For this review, take the finished solid that the model builds, in its own axes (mm). A direction names the side the tool comes from. Give positions to 0.01 mm unless a question says otherwise; leave off trailing zeros. Write each loop counter-clockwise with the first axis right and the second up, starting at its lowest first coordinate (ties: lowest second). Pieces come first, ordered by that corner, then holes.
1) We need section D-D on x = 2.5. Give the boundary of the cut face in (y, z), and give its area (3 significant figures).
2) Draft analysis for pull direction X (two halves, no side actions). For faces 3 (the face through (-9.613, 3.514, 23.186)), 4 (the face through (-27.07, 2.28, 27)), 5 (the face through (0, 3, 28.5)), state which applies: pulls with the +X half, pulls with the -X half, needs draft (parallel to the pull), parting line crosses it, or undercut.
3) We need section B-B on z = 18. Give the boundary of the cut face in (x, y).
4) We need section C-C on y = 3.5. Give the number of separate pieces and of enclosed holes in the cut face, and give its area (3 significant figures).
5) We need section A-A on x = 22. Give the boundary of the cut face in (y, z).
6) For P1, Ø6.5, axis at x = 23.5, z = -23.5, coming from the +Y side, flat-tipped, find the tip position at first contact; note if it passes through.
7) Machinability: for faces 1 (the face through (15.88, 1.27, -17.32)), 2 (the face through (22.4, 2.5, -7.6)), which of the approach directions +Z, -Z, +X, -X, +Y, -Y give a long, thin tool a straight path to every point of the face, cutting with its end or side? Answer none if there is none.
8) Wall thickness on line 1 along X through (y, z) = (1.15, 0); line 2 along X through (y, z) = (3.55, 15.5); line 3 along Y through (x, z) = (-5, 26.5): over which ranges is each line inside the solid? List them lowest first.
from build123d import *

# Parameters (mm, degrees)
SKETCH1_W                = 57
SKETCH1_H                = 57
BOSS_EXTRUDE1_DEPTH      = 4.5
FILLET1_R                = 5
SKETCH2_R                = 2.5
SKETCH2_R_2              = 1.7
CUT_EXTRUDE1_DEPTH       = 41.555517504
BOSS_EXTRUDE2_DEPTH      = 1
FILLET2_R                = 0.2
SKETCH4_R                = 23.5
CUT_EXTRUDE2_DEPTH       = 41.555517504
SKETCH4_3_R              = 25.1
SKETCH4_3_R_2            = 23.5
CUT_EXTRUDE3_DEPTH       = 2
CUT_EXTRUDE4_DEPTH       = 1.1
CIRPATTERN1_COUNT        = 4
FILLET2_OF_CIRPATTERN1_R = 0.2


with BuildPart() as part:
    # Sketch1 → Boss-Extrude1 (new body)
    with BuildSketch(Plane(origin=(0, 0, 0), x_dir=(1, 0, 0), z_dir=(0, 1, 0))):
        Rectangle(SKETCH1_W, SKETCH1_H)
    extrude(amount=BOSS_EXTRUDE1_DEPTH)

    # Fillet1
    fillet1_edges = [part.edges().sort_by_distance(p)[0] for p in [
        (-28.5, 2.25, -28.5),
        (28.5, 2.25, -28.5),
        (28.5, 2.25, 28.5),
        (-28.5, 2.25, 28.5),
    ]]
    fillet(fillet1_edges, radius=FILLET1_R)

    # Sketch2 → Cut-Extrude1 (cut, through all)
    with BuildSketch(Plane(origin=(0, 4.5, 0), x_dir=(1, 0, 0), z_dir=(0, 1, 0))):
        with Locations(Location((-23.5, 23.5, 0), (0, 0, 270))):
            Circle(SKETCH2_R)
        with Locations(Location((-15.5, 25, 0), (0, 0, 270))):
            Circle(SKETCH2_R_2)
    cut_extrude1 = extrude(amount=-CUT_EXTRUDE1_DEPTH, mode=Mode.SUBTRACT)

    # Sketch3 → Boss-Extrude2 (add)
    with BuildSketch(Plane(origin=(0, 4.5, 0), x_dir=(1, 0, 0), z_dir=(0, 1, 0))):
        Polygon((11, 27.5), (-11, 27.5), (-12, 28.5), (12, 28.5), align=None)
    boss_extrude2 = extrude(amount=BOSS_EXTRUDE2_DEPTH)

    # Fillet2
    fillet2_edges = [part.edges().sort_by_distance(p)[0] for p in [
        (0, 5.5, -27.5),
    ]]
    fillet(fillet2_edges, radius=FILLET2_R)

    # Sketch4 → Cut-Extrude2 (cut, through all)
    with BuildSketch(Plane(origin=(0, 4.5, 0), x_dir=(1, 0, 0), z_dir=(0, 1, 0))):
        with Locations(Location((0, 0, 0), (0, 0, 270))):
            Circle(SKETCH4_R)
    extrude(amount=-CUT_EXTRUDE2_DEPTH, mode=Mode.SUBTRACT)

    # Sketch4_3 → Cut-Extrude3 (cut)
    with BuildSketch(Plane(origin=(0, 4.5, 0), x_dir=(1, 0, 0), z_dir=(0, 1, 0))):
        with Locations(Location((0, 0, 0), (0, 0, 270))):
            Circle(SKETCH4_3_R)
        with Locations(Location((0, 0, 0), (0, 0, 270))):
            Circle(SKETCH4_3_R_2, mode=Mode.SUBTRACT)
    extrude(amount=-CUT_EXTRUDE3_DEPTH, mode=Mode.SUBTRACT)

    # Sketch5 → Cut-Extrude4 (cut)
    with BuildSketch(Plane.XZ):
        Polygon((-11, -27.5), (11, -27.5), (12, -28.5), (-12, -28.5), align=None)
    cut_extrude4 = extrude(amount=-CUT_EXTRUDE4_DEPTH, mode=Mode.SUBTRACT)

    # CirPattern1: Cut-Extrude1, Boss-Extrude2, Cut-Extrude4 ×4 about axis
    cirpattern1_axis = Axis((0, 0, 0), (0, 1, 0))
    add([cut_extrude1.rotate(cirpattern1_axis, i * 360 / CIRPATTERN1_COUNT) for i in range(1, CIRPATTERN1_COUNT)], mode=Mode.SUBTRACT)
    add([boss_extrude2.rotate(cirpattern1_axis, i * 360 / CIRPATTERN1_COUNT) for i in range(1, CIRPATTERN1_COUNT)])
    add([cut_extrude4.rotate(cirpattern1_axis, i * 360 / CIRPATTERN1_COUNT) for i in range(1, CIRPATTERN1_COUNT)], mode=Mode.SUBTRACT)

    # Fillet2 of CirPattern1
    fillet2_of_cirpattern1_edges = [part.edges().sort_by_distance(p)[0] for p in [
        (-27.5, 5.5, 0),
        (0, 5.5, 27.5),
        (27.5, 5.5, 0),
    ]]
    fillet(fillet2_of_cirpattern1_edges, radius=FILLET2_OF_CIRPATTERN1_R)


solid = part.part
Results list:
1. outline: (0, -27.5) - (1.1, -27.5) - (1.1, -28.5) - (5.5, -28.5) - (5.5, -27.7) arc R0.2 ccw to (5.3, -27.5) - (4.5, -27.5) - (4.5, -24.98) - (2.5, -24.98) - (2.5, -23.37) - (0, -23.37) - close; (0, 23.37) - (2.5, 23.37) - (2.5, 24.98) - (4.5, 24.98) - (4.5, 27.5) - (5.3, 27.5) arc R0.2 ccw to (5.5, 27.7) - (5.5, 28.5) - (1.1, 28.5) - (1.1, 27.5) - (0, 27.5) - close
1. area: 39.5 mm2
2. face 3: undercut
2. face 4: pulls with the -X half
2. face 5: needs draft
3. outline: (-28.5, 0) - (-15.11, 0) - (-15.11, 2.5) - (-17.49, 2.5) - (-17.49, 4.5) - (-28.5, 4.5) - close; (15.11, 0) - (28.5, 0) - (28.5, 4.5) - (17.49, 4.5) - (17.49, 2.5) - (15.11, 2.5) - close
4. separate pieces: 1
4. enclosed holes: 9
4. area: 1,130 mm2
5. outline: (0, -28.5) - (4.5, -28.5) - (4.5, -25.5) - (0, -25.5) - close; (0, -21.5) - (4.5, -21.5) - (4.5, -12.08) - (2.5, -12.08) - (2.5, -8.26) - (0, -8.26) - close; (0, 8.26) - (2.5, 8.26) - (2.5, 12.08) - (4.5, 12.08) - (4.5, 21.5) - (0, 21.5) - close; (0, 25.5) - (4.5, 25.5) - (4.5, 28.5) - (0, 28.5) - close
6. P1: stops at y = 4.5
7. face 1: +Y, -Y
7. face 2: +Y
8. line 1: x = -28.5 to -23.5, 23.5 to 28.5
8. line 2: x = -28.5 to -26.7, -23.3 to -19.74, 19.74 to 28.5
8. line 3: y = 0 to 4.5
